Here's how the part is built. I have some questions about the finished solid (model axes, mm). Face numbers are marked on the shaded views. A direction names the side the tool comes from. Coordinates: 2 decimals unless noted, no trailing zeros. Write each loop counter-clockwise with the first axis right and the second up, starting at its lowest first coordinate (ties: lowest second). Pieces come first, ordered by that corner, then holes.
Item 1: I want a section at A-A (z = -38). Please give me the cut outline in (x, y).
Item 2: For the marked faces 1 and 2, which set-ups out of +Z, -Z, +X, -X, +Y, -Y let a thin tool reach every point of the face, with its end or its side?
Item 3: I want a section at B-B (x = 13). Please give me the cut outline in (y, z).
Item 4: I want a section at D-D (z = -4.5). Please give me the cut outline in (x, y).
Item 5: Please list where these lines run through material, in increasing order: line 1 (X direction, y = 3.2, z = -38); line 2 (Y direction, x = 36.5, z = -10.5); line 3 (X direction, y = 4.1, z = -36.5).
Item 6: I want a section at C-C (x = 26.5). Please give me the cut outline in (y, z), and give its area (3 significant figures).
Item 7: I'm going to push flat-ended pins straight in: P1, Ø3, axis at x = 28, z = -63.5, coming from the -Y side; P2, Ø0.9, axis at x = 4, z = -47.5, coming from the +Y side; P3, Ø4, axis at x = 42, z = -15.5, coming from the +Y side; P4, Ø9, axis at x = 13, z = -38, coming from the -Y side. Where does each tip first touch, or does it pass through?
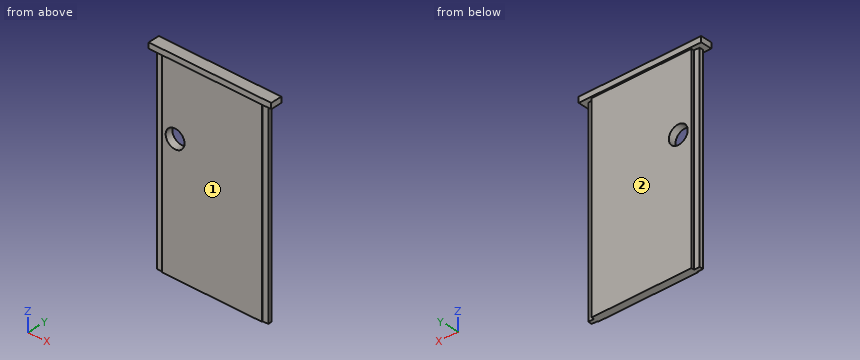
from build123d import *

# Parameters (mm, degrees)
SKETCH1_W           = 65
SKETCH1_H           = 6
BOSS_EXTRUDE1_DEPTH = 3
SKETCH2_W           = 53
SKETCH2_H           = 4
SKETCH2_W_2         = 3
SKETCH2_H_2         = 2
BOSS_EXTRUDE2_DEPTH = 105
SKETCH3_R           = 5
CUT_EXTRUDE1_DEPTH  = 98


with BuildPart() as part:
    # Sketch1 → Boss-Extrude1 (new body)
    with BuildSketch(Plane.XY):
        with Locations((32.5, 3)):
            Rectangle(SKETCH1_W, SKETCH1_H)
    extrude(amount=BOSS_EXTRUDE1_DEPTH)

    # Sketch2 → Boss-Extrude2 (add)
    with BuildSketch(Plane(origin=(0, 0, 0), x_dir=(-1, 0, 0), z_dir=(0, 0, -1))):
        with Locations((-32.5, 3.1)):
            Rectangle(SKETCH2_W, SKETCH2_H)
        with Locations((-60.5, 2.6)):
            Rectangle(SKETCH2_W_2, SKETCH2_H_2)
        with Locations((-4.5, 2.6)):
            Rectangle(SKETCH2_W_2, SKETCH2_H_2)
    extrude(amount=BOSS_EXTRUDE2_DEPTH)

    # Sketch3 → Cut-Extrude1 (cut)
    with BuildSketch(Plane(origin=(0, 5.1, 0), x_dir=(1, 0, 0), z_dir=(0, 1, 0))):
        with Locations(Location((13, 38, 0), (0, 0, 270))):
            Circle(SKETCH3_R)
    extrude(amount=-CUT_EXTRUDE1_DEPTH, mode=Mode.SUBTRACT)


solid = part.part
Answer:
1. outline: (3, 1.6) - (6, 1.6) - (6, 1.1) - (8, 1.1) - (8, 5.1) - (6, 5.1) - (6, 3.6) - (3, 3.6) - close; (18, 1.1) - (59, 1.1) - (59, 1.6) - (62, 1.6) - (62, 3.6) - (59, 3.6) - (59, 5.1) - (18, 5.1) - close
2. face 1: -Z, +X, -X, -Y
2. face 2: -Z, +X, -X, +Y
3. outline: (0, 0) - (1.1, 0) - (1.1, -33) - (5.1, -33) - (5.1, 0) - (6, 0) - (6, 3) - (0, 3) - close; (1.1, -105) - (5.1, -105) - (5.1, -43) - (1.1, -43) - close
4. outline: (3, 1.6) - (6, 1.6) - (6, 1.1) - (59, 1.1) - (59, 1.6) - (62, 1.6) - (62, 3.6) - (59, 3.6) - (59, 5.1) - (6, 5.1) - (6, 3.6) - (3, 3.6) - close
5. line 1: x = 3 to 8, 18 to 62
5. line 2: y = 1.1 to 5.1
5. line 3: x = 6 to 8.23, 17.77 to 59
6. outline: (0, 0) - (1.1, 0) - (1.1, -105) - (5.1, -105) - (5.1, 0) - (6, 0) - (6, 3) - (0, 3) - close
6. area: 438 mm2
7. P1: stops at y = 1.1
7. P2: stops at y = 3.6
7. P3: stops at y = 5.1
7. P4: passes through
